Geometry: final body of the model. Coordinates: model frame, mm. Face numbers are marked on the shaded views. A direction names the side the tool comes from. Coordinates: 2 decimals unless noted, no trailing zeros. Loops run counter-clockwise (first coordinate to the right, second up) from the corner with the lowest first, then second, coordinate; pieces in that order, holes last. Notation, with made-up numbers: (-35, 36) -> (-19, 36) arc R31 ccw to (-19, 69) -> close; hole circle Ø3 at (-22.75, -17.5). An arc over 180 degrees is marked (long way). One line per item, written item: value. Start each with the question number.
Item 1: Set-up query: the marked faces 5, 6 and 7. Return all of +Z, -Z, +X, -X, +Y, -Y with unobstructed straight access to the full face (end or side cutting, diameter ignored); none if empty.
Item 2: Ray query, probe 1 along Y at (x, z) = (17.75, -97.5); probe 2 along Z at (x, y) = (3.75, -15); probe 3 along Z at (x, y) = (14.5, -6). Return the intervals inside material, ascending. Write a range as from..to.
Item 3: Section query D-D on y = -17. Return loops of the section in (x, z).
Item 4: Contact query for flat-ended pins moving along their axis: pin 1 Ø10 at (y, z) = (8, -41.5) entering from +X; pin 2 Ø2 at (x, z) = (8, -25) entering from +Y; pin 3 Ø5 at (y, z) = (-3.5, -32.5) entering from -X; pin 4 Ø10 at (x, z) = (14, -43.5) entering from -Y. Output: stop coordinate, or through.
Item 5: Section query A-A on x = 3. Return loops of the section in (y, z) (1 decimal), then the cut area to 3 significant figures.
Item 6: Section query C-C on z = -85.5. Return loops of the section in (x, y).
Item 7: Section query B-B on y = -2.5. Return loops of the section in (x, z), then the cut area to 3 significant figures.
Item 8: Mould query, pull axis Z, two halves, no side actions, for the marked faces 1, 2, 3 and 4. Classes: +Z half, -Z half, draft (parallel to the pull), parting line (faces both ways), or undercut.
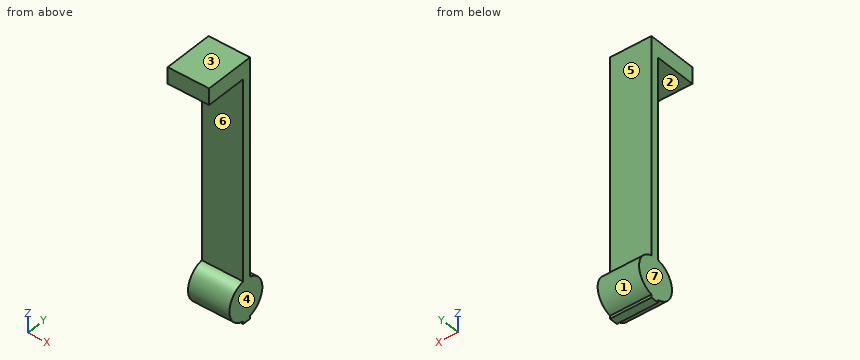
Autodesk Inventor part; units mm, degrees
ref_plane "YZ Plane" through (0, 0, 0) normal (1, 0, 0) x (0, 1, 0)
ref_plane "XZ Plane" through (0, 0, 0) normal (0, 1, 0) x (-1, 0, 0)
ref_plane "XY Plane" through (0, 0, 0) normal (0, 0, 1) x (1, 0, 0)
sketch "Эскиз1" plane through (0, 0, 0) normal (1, 0, 0) x (0, 1, 0)
  line L0 (0, 0) -> (4, 0)
  line L1 (4, 0) -> (4, -125)
  line L2 (4, -125) -> (0, -125)
  line L3 (0, -125) -> (0, 0)
  dimension "d0" = 4
  dimension "d1" = 125
extrude "Выдавливание1" add sketch "Эскиз1" along normal blind 20
sketch "Эскиз3" plane through (20, 0, 0) normal (1, 0, 0) x (0, 0, -1)
  circle A0 centre (114.225, 1.5875) radius 9.6564
  line L0 (125, 0) -> (125, 4)
  point P0 (0, 0)
  dimension "d8" = 10.775
extrude "Выдавливание3" add sketch "Эскиз3" against normal blind 20
sketch "Эскиз5" plane through (0, 0, 0) normal (0, -1, 0) x (1, 0, 0)
  line L0 (20, -104.8748) -> (20, 0)
  line L1 (0, 0) -> (20, 0)
  line L2 (20, 0) -> (20, -7.9375)
  line L3 (20, -7.9375) -> (0, -7.9375)
  line L4 (0, -7.9375) -> (0, 0)
extrude "Выдавливание5" add sketch "Эскиз5" along normal blind 20
properties part number "ПАЛЬЧИК"
Reply:
1. face 5: +Z, +X, -X, +Y
1. face 6: +X, -X, -Y
1. face 7: +Z, -Z, -X, +Y, -Y
2. probe 1: y = 0..4
2. probe 2: z = -7.94..0
2. probe 3: z = -120.2..-108.25, -7.94..0
3. outline: (0, -7.94) -> (20, -7.94) -> (20, 0) -> (0, 0) -> close
4. pin 1: stops at x = 20
4. pin 2: stops at y = 4
4. pin 3: passes through
4. pin 4: stops at y = 0
5. outline: (-20, -7.9) -> (0, -7.9) -> (0, -104.7) arc R9.7 ccw to (0, -123.8) -> (0, -125) -> (4, -125) -> (4, -123.6) arc R9.7 ccw to (4, -104.9) -> (4, 0) -> (-20, 0) -> close
5. area: 875 mm²
6. outline: (0, 0) -> (20, 0) -> (20, 4) -> (0, 4) -> close
7. outline: (0, -122.97) -> (20, -122.97) -> (20, -105.48) -> (0, -105.48) -> close; (0, -7.94) -> (20, -7.94) -> (20, 0) -> (0, 0) -> close
7. area: 509 mm²
8. face 1: parting line
8. face 2: undercut
8. face 3: +Z half
8. face 4: draft
